Verification items for the finished model (mm, model axes). Face numbers are marked on the shaded views. A direction names the side the tool comes from. Give positions to 0.01 mm unless a question says otherwise; leave off trailing zeros. Write each loop counter-clockwise with the first axis right and the second up, starting at its lowest first coordinate (ties: lowest second). Pieces come first, ordered by that corner, then holes. Notation, with made-up numbers: (-26, 46) -> (-8, 46) arc R11 ccw to (-8, 52) -> close; hole circle Ø5 at (25, 51.25). An arc over 180 degrees is marked (long way). Answer as CSV lines item,"result". Start each with the question number.
1) Gauge pin test, flat ends, axial feed: pin 1 Ø0.6 at (x, z) = (3, 0.5) entering from +Y; pin 2 Ø1 at (x, z) = (-6.5, 16) entering from +Y; pin 3 Ø12 at (x, y) = (-1, 13) entering from +Z. Record the tip position at first contact, or that the pin passes through.
2) Tool access check on the marked faces 1 and 2. Record the directions out of +Z, -Z, +X, -X, +Y, -Y that give a thin tool (end or side, any length) a straight path to the whole face; none if there is none.
3) Material ranges on L1, parallel to Z at x = 1, y = -25; L2, parallel to Y at x = -11.5, z = 4.25; L3, parallel to Y at x = 7.5, z = 3.75, recorded low to high.
4) Mould release check, pull along Y, two halves, no side actions. Record for the marked faces 3, 4 and 5: released by +Y, released by -Y, zero draft, split by the parting line, or undercut.
5) Sectioned sample at B-B on y = -26.5. Record the cut outline in (x, z).
6) Sectioned sample at D-D on y = 9. Record the cut outline in (x, z).
7) Sectioned sample at C-C on z = 12.5. Record the cut outline in (x, y), and give its area (3 significant figures).
```python
from build123d import *

# Parameters (mm, degrees)
F1_DEPTH    = 13.25
F2_DEPTH    = 13.25
F3_R        = 1.99999
F4_R        = 2
F5_T1_DEPTH = 26.5


# Not quite as in the source:
# - a fillet or chamfer that OpenCascade refuses, or shapes differently, is made with other operations: its cross-section is extruded or revolved along the edge and cut away or added
# - a fillet or chamfer is up to 0.001 mm smaller than in the source, because OpenCascade refuses the exact size
# - a feature names something its author has since deleted; it is built from what else it names


with BuildPart() as f1:
    # F0 (on Right) → F1 (new body, symmetric)
    with BuildSketch(Plane.YZ):
        with BuildLine():
            Line((24.6479697927, -2.219830174), (-24.9527402653, 20.909360776))
            Line((-24.9527402653, 20.909360776), (-27.4884498358, 15.4715140538))
            Line((-27.4884498358, 15.4715140538), (-23.8632186876, 13.7810410068))
            Line((-23.8632186876, 13.7810410068), (-23.0179821641, 15.5936565809))
            Line((-23.0179821641, 15.5936565809), (5.077559234, 2.4924904669))
            Line((5.077559234, 2.4924904669), (7.7964825951, 1.2246356817))
            Line((7.7964825951, 1.2246356817), (15.1652631053, -2.2114831015))
            Line((15.1652631053, -2.2114831015), (5.077559234, -2.2175114543))
            Line((5.077559234, -2.2175114543), (1.1974681402, -2.219830174))
            Line((1.1974681402, -2.219830174), (-27.1520302073, -2.219830174))
            Line((-27.1520302073, -2.219830174), (-27.1520302073, 1.780169826))
            Line((-27.1520302073, 1.780169826), (-30.3520302073, 1.780169826))
            Line((-30.3520302073, 1.780169826), (-30.3520302073, -6.219830174))
            Line((-30.3520302073, -6.219830174), (24.6479697927, -6.219830174))
            ThreePointArc((24.6479697927, -6.219830174), (25.9221103143, -4.219830174), (24.6479697927, -2.219830174))
        make_face()
        with BuildLine():
            Line((-23.8632186876, 13.7810410068), (-27.4884498358, 15.4715140538))
            ThreePointArc((-27.4884498358, 15.4715140538), (-29.6284726398, 8.7739706401), (-30.3520302073, 1.780169826))
            Line((-30.3520302073, 1.780169826), (-27.1520302073, 1.780169826))
            ThreePointArc((-27.1520302073, 1.780169826), (-26.3149438564, 8.0018494688), (-23.8632186876, 13.7810410068))
        make_face()
        Polygon((7.7964825951, 1.2246356817), (5.077559234, 2.4924904669), (5.077559234, -2.2175114543), (15.1652631053, -2.2114831015), align=None)
    extrude(amount=F1_DEPTH, both=True)

    # F0 (on Right) → F2 (join, symmetric)
    with BuildSketch(Plane.YZ):
        with BuildLine():
            Line((24.6479697927, -2.219830174), (-24.9527402653, 20.909360776))
            Line((-24.9527402653, 20.909360776), (-27.4884498358, 15.4715140538))
            Line((-27.4884498358, 15.4715140538), (-23.8632186876, 13.7810410068))
            Line((-23.8632186876, 13.7810410068), (-23.0179821641, 15.5936565809))
            Line((-23.0179821641, 15.5936565809), (5.077559234, 2.4924904669))
            Line((5.077559234, 2.4924904669), (7.7964825951, 1.2246356817))
            Line((7.7964825951, 1.2246356817), (15.1652631053, -2.2114831015))
            Line((15.1652631053, -2.2114831015), (5.077559234, -2.2175114543))
            Line((5.077559234, -2.2175114543), (1.1974681402, -2.219830174))
            Line((1.1974681402, -2.219830174), (-27.1520302073, -2.219830174))
            Line((-27.1520302073, -2.219830174), (-27.1520302073, 1.780169826))
            Line((-27.1520302073, 1.780169826), (-30.3520302073, 1.780169826))
            Line((-30.3520302073, 1.780169826), (-30.3520302073, -6.219830174))
            Line((-30.3520302073, -6.219830174), (24.6479697927, -6.219830174))
            ThreePointArc((24.6479697927, -6.219830174), (25.9221103143, -4.219830174), (24.6479697927, -2.219830174))
        make_face()
    extrude(amount=F2_DEPTH, both=True)

    # F3 (radius 2 in the source; OpenCascade refuses exactly that, so slightly less here)
    f3_edges = [f1.edges().sort_by_distance(p)[0] for p in [
        (0, -23.017982, 15.593657),
        (0, 24.64797, -2.21983),
        (0, 24.64797, -6.21983),
    ]]
    fillet(f3_edges, radius=F3_R)

    # F4
    f4_edges = [f1.edges().sort_by_distance(p)[0] for p in [
        (0, -27.15203, -2.21983),
        (0, -30.35203, -6.21983),
        (0, -30.35203, 1.78017),
    ]]
    fillet(f4_edges, radius=F4_R)

    # F5: fillet of radius 3 on 2 edges, made by hand

    # F5_s2 → F5_t1 (join)
    with BuildSketch(Plane.YZ.offset(-13.25)):
        with BuildLine():
            ThreePointArc((2.0793520161, -2.2193031654), (4.1995133271, -1.3399901057), (5.077559234, 0.780696299))
            Line((5.077559234, 0.780696299), (5.077559234, -2.2175114543))
            Line((5.077559234, -2.2175114543), (2.0793520161, -2.2193031654))
        make_face()
        with BuildLine():
            ThreePointArc((5.077559234, 0.5812796845), (4.6077335715, 2.1931785095), (3.3454140192, 3.3002030456))
            Line((3.3454140192, 3.3002030456), (5.077559234, 2.4924904669))
            Line((5.077559234, 2.4924904669), (5.077559234, 0.5812796845))
        make_face()
    extrude(amount=F5_T1_DEPTH)


solid = f1.part
```
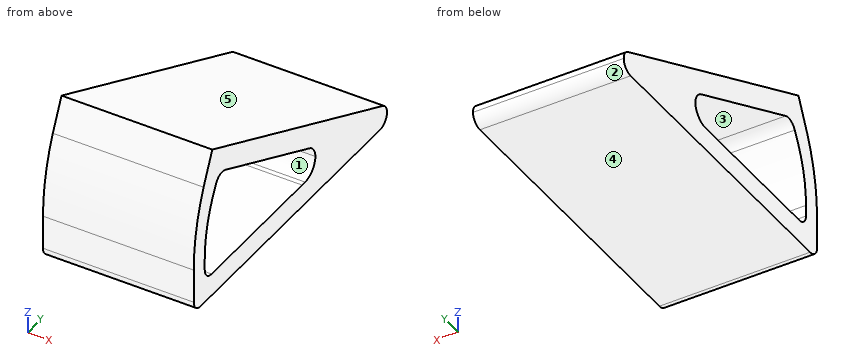
Ans:
1,pin 1,"stops at y = 19.46"
1,pin 2,"stops at y = -13.35"
1,pin 3,"stops at z = 6.01"
2,face 1,"+X, -X"
2,face 2,"-Z, +X, -X, +Y"
3,L1,"z = -6.22 to -2.22, 11.61 to 20.81"
3,L2,"y = -30.26 to -27.02, 1.31 to 10.77"
3,L3,"y = -30.3 to -27.07, 2.38 to 11.85"
4,face 3,"undercut"
4,face 4,"zero draft"
4,face 5,"released by +Y"
5,outline,"(-13.25, -6.22) -> (13.25, -6.22) -> (13.25, -1.7) -> (-13.25, -1.7) -> close; (-13.25, 7.28) -> (13.25, 7.28) -> (13.25, 17.59) -> (-13.25, 17.59) -> close"
6,outline,"(-13.25, -6.22) -> (13.25, -6.22) -> (13.25, 5.08) -> (-13.25, 5.08) -> close"
7,outline,"(-13.25, -28.63) -> (13.25, -28.63) -> (13.25, -24.57) -> (-13.25, -24.57) -> close; (-13.25, -16.38) -> (13.25, -16.38) -> (13.25, -6.92) -> (-13.25, -6.92) -> close"
7,area,"358 mm²"
